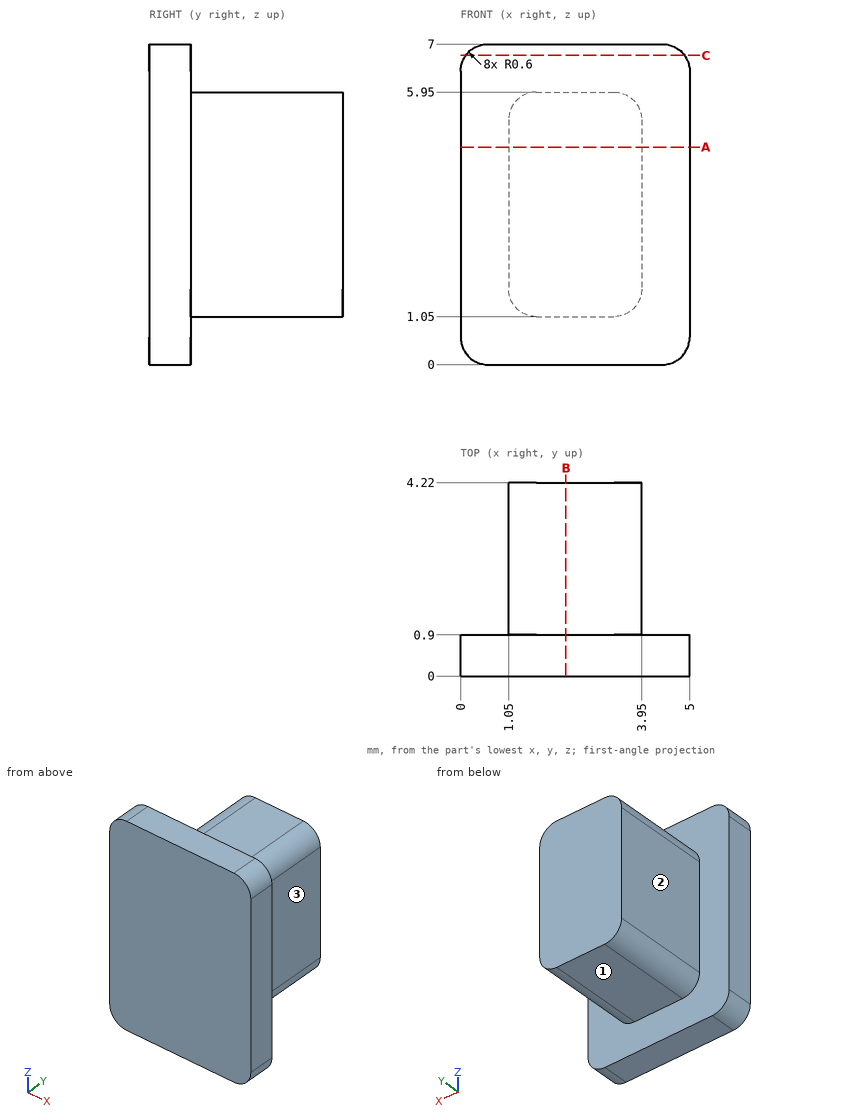
Design review of the part shown in the three views and the two pictorial views. Dimensions are in mm from the part's minimum x, y and z. A direction names the side the tool comes from. Coordinates: 2 decimals unless noted, no trailing zeros. Order: outer loops, then holes, each group sorted by start corner. A loop starts at its lowest first (then second) coordinate and runs counter-clockwise, first axis right, second up.
1) Clearance check with flat-ended pins moving along their axes: pin 1 (0.5 mm diameter, centred on x = 2.5, y = 3, fed in from +Z); pin 2 (1.9 mm diameter, centred on x = 3, y = 2.5, fed in from -Z); pin 3 (1.7 mm diameter, centred on y = 3, z = 3, fed in from -X). State where each tip first meets the part, or that it passes through.
2) Take a section at B-B, the plane x = 2.3. Give the boundary of the cut face in (y, z), and give its area (3 significant figures).
3) Take a section at A-A, the plane z = 4.75. Give the boundary of the cut face in (x, y), and give its area (3 significant figures).
4) Take a section at C-C, the plane z = 6.75. Give the boundary of the cut face in (x, y), and give its area (3 significant figures).
5) Wall thickness on line 1 along Z through (x, y) = (1.95, 2.6); line 2 along X through (y, z) = (2.9, 4.75); line 3 along Y through (x, z) = (0.85, 2.5): over which ranges is each line inside the solid? List them lowest first.
6) For the marked faces 1, 2 and 3, list the 3-axis set-ups (+Z, -Z, +X, -X, +Y, -Y) from which the entire face can be reached by the end or side of a thin tool; tool diameter is ignored.
Returned:
1. pin 1: stops at z = 5.95
1. pin 2: stops at z = 1.05
1. pin 3: stops at x = 1.05
2. outline: (0, 0) - (0.9, 0) - (0.9, 1.05) - (4.22, 1.05) - (4.22, 5.95) - (0.9, 5.95) - (0.9, 7) - (0, 7) - close
2. area: 22.6 mm2
3. outline: (0, 0) - (5, 0) - (5, 0.9) - (3.95, 0.9) - (3.95, 4.22) - (1.05, 4.22) - (1.05, 0.9) - (0, 0.9) - close
3. area: 14.1 mm2
4. outline: (0.11, 0) - (4.89, 0) - (4.89, 0.9) - (0.11, 0.9) - close
4. area: 4.30 mm2
5. line 1: z = 1.05 to 5.95
5. line 2: x = 1.05 to 3.95
5. line 3: y = 0 to 0.9
6. face 1: -Z, +X, -X, +Y
6. face 2: +Z, -Z, -X, +Y
6. face 3: +Z, -Z, +X, +Y
